Geometry check sheet. Reference: drawing and pictorial views, mm from the part's lowest x, y, z. Coordinates: 2 decimals unless noted, no trailing zeros. Write each loop counter-clockwise with the first axis right and the second up, starting at its lowest first coordinate (ties: lowest second). Pieces come first, ordered by that corner, then holes. Notation, with made-up numbers: M 65.5,45 L 120.5,45 A23 ccw 120.5,57 Z; hole C -38,-4 d11. An arc over 180 degrees is marked long. One line per item, written item: value.
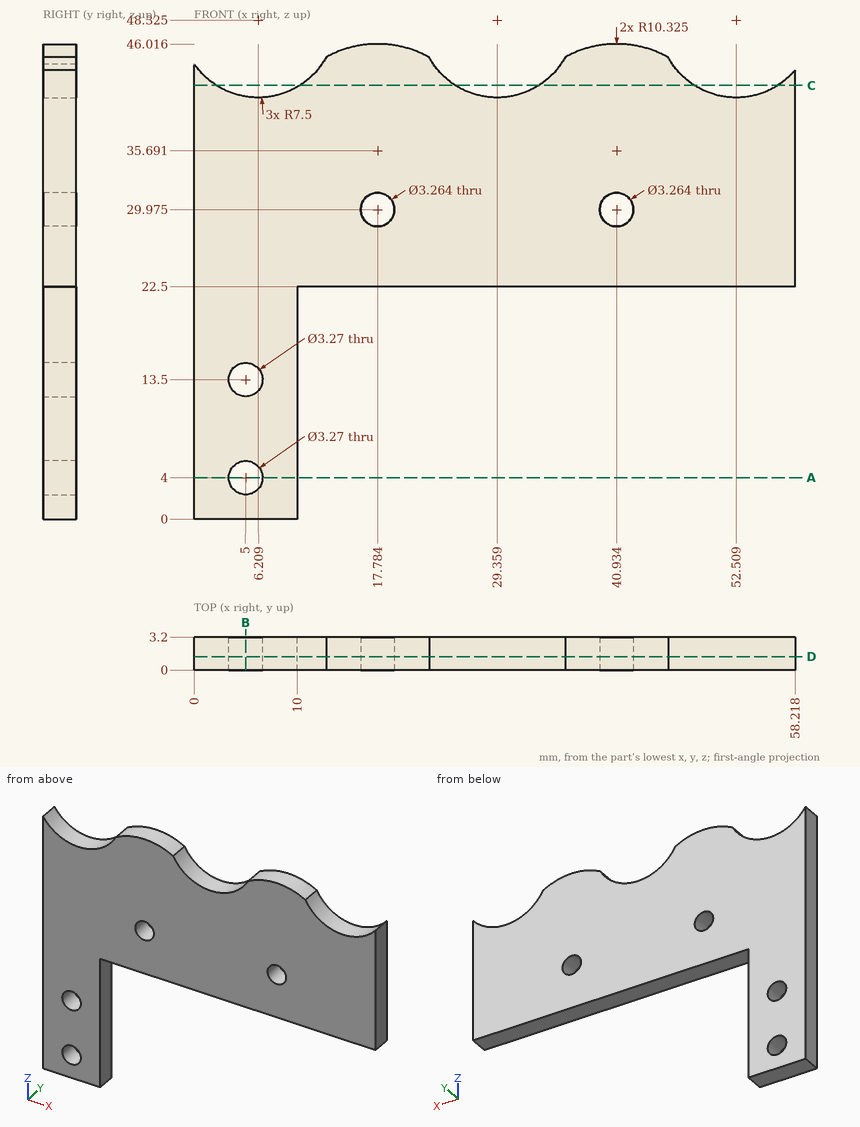
Item 1: Cross-section at D-D, the plane y = 1.3. Give the number of separate pieces and of enclosed holes in the cut face, and give its area (3 significant figures).
The answers:
separate pieces: 1
enclosed holes: 4
area: 1,390 mm²
Item 2: Cross-section at B-B, the plane x = 5. Enter the section's corners in (y, z) (3 decimals), and give its area (3 significant figures).
The answers:
outline: M 0,0 L 3.2,0 L 3.2,2.365 L 0,2.365 Z; M 0,5.635 L 3.2,5.635 L 3.2,11.865 L 0,11.865 Z; M 0,15.135 L 3.2,15.135 L 3.2,40.923 L 0,40.923 Z
area: 110 mm²
Item 3: Go/stop test with flat-tipped pins: P1, Ø2.5, axis at x = 5, z = 13.5, coming from the -Y side (3 decimals); P2, Ø1.6, axis at y = 1.5, z = 6, coming from the +X side; P3, Ø1, axis at x = 35, y = 1.5, coming from the +Z side; P4, Ø1, axis at x = 26.5, y = 0.5, coming from the +Z side. Record where each tip stops, or that it passes through.
The answers:
P1: passes through
P2: stops at x = 10
P3: stops at z = 44.02
P4: stops at z = 41.62
Item 4: Scan lines: line 1 (X direction, y = 2.25, z = 13.5) (3 decimals); line 2 (Z direction, x = 41.5, y = 0.55); line 3 (X direction, y = 1.6, z = 18). Record each from-to range of solid material in increasing order.
The answers:
line 1: x = 0 to 3.365, 6.635 to 10
line 2: z = 22.5 to 28.44, 31.51 to 46
line 3: x = 0 to 10
Item 5: Cross-section at C-C, the plane z = 42. Enter the section's corners in (x, y).
The answers:
outline: M 0,0 L 2.18,0 L 2.18,3.2 L 0,3.2 Z; M 10.24,0 L 25.33,0 L 25.33,3.2 L 10.24,3.2 Z; M 33.39,0 L 48.48,0 L 48.48,3.2 L 33.39,3.2 Z; M 56.54,0 L 58.22,0 L 58.22,3.2 L 56.54,3.2 Z
Item 6: Cross-section at A-A, the plane z = 4. Enter the section's corners in (x, y) (3 decimals).
The answers:
outline: M 0,0 L 3.365,0 L 3.365,3.2 L 0,3.2 Z; M 6.635,0 L 10,0 L 10,3.2 L 6.635,3.2 Z
